```python
from build123d import *

# Parameters (mm, degrees)
F2_R     = 2
F3_DEPTH = 3
F4_R     = 1.5
F5_DEPTH = 8
F6_SIZE  = 0.2


with BuildPart() as f1:
    # F0 (on Right) → F1 (revolve)
    with BuildSketch(Plane.YZ):
        with BuildLine():
            Line((0, 3.25), (0, -3.25))
            ThreePointArc((0, -3.25), (3.25, 0), (0, 3.25))
        make_face()
    revolve(axis=Axis((0, 0, 0), (0, 0, -1)))

    # F2 (on Top) → F3 (join)
    with BuildSketch(Plane.XY):
        Circle(F2_R)
    extrude(amount=F3_DEPTH)

    # F4 (on face) → F5 (join)
    with BuildSketch(Plane.XY.offset(3)):
        Circle(F4_R)
    extrude(amount=F5_DEPTH)

    # F6
    f6_edges = [f1.edges().sort_by_distance(p)[0] for p in [
        (-1.5, 0, 11),
    ]]
    chamfer(f6_edges, length=F6_SIZE)


solid = f1.part
```
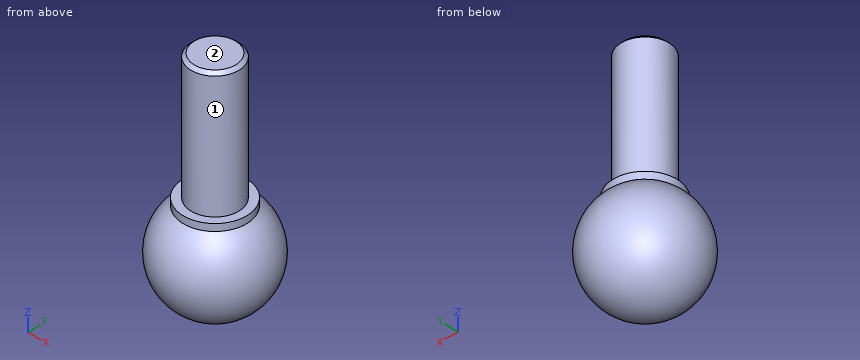
CAD build for the part. Positions are in the model's coordinates, mm. Face numbers are marked on the shaded views. A direction names the side the tool comes from. Give positions to 0.01 mm unless a question says otherwise; leave off trailing zeros. Write each loop counter-clockwise with the first axis right and the second up, starting at its lowest first coordinate (ties: lowest second). Pieces come first, ordered by that corner, then holes. Notation, with made-up numbers: M 69,21.5 L 113,21.5 A11 cw 113,29.5 Z; hole C 24,89 d7. An arc over 180 degrees is marked long. Return JSON: item names as keys, results as strings. Group by question number.
(1) 3-axis set-ups, long thin cutter, end or side, ignore diameter. For the marked faces 1 and 2: which of +Z, -Z, +X, -X, +Y, -Y reach the whole face in a straight line?
(2) Flat gauge pins, fed straight in: pin 1 Ø2 at (x, z) = (2, 9) entering from +Y; pin 2 Ø2 at (x, y) = (0, 1.5) entering from +Z. Where does each tip first touch, or does it go through?
(3) Band-saw the part on A-A (y = 0). Give the cut face in (x, z).
(4) Band-saw the part on D-D (z = 3.5). Give the cut face in (x, y).
(5) Band-saw the part on C-C (z = 1.25). Give the cut face in (x, y).
(6) Drill centre lines: L1, parallel to X at y = -0.25, z = 1.25; L2, parallel to X at y = 1, z = 2.75; L3, parallel to Y at x = 2, z = -2. Where is each one in solid material? Low to high. Write a range as [from, to].
Entries:
{
 "1": {"face 1": "+Z", "face 2": "+Z, +X, -X, +Y, -Y"},
 "2": {"pin 1": "stops at y = 1.12", "pin 2": "stops at z = 11"},
 "3": {"outline": "M -2,2.56 A3.25 ccw long 2,2.56 L 2,3 L 1.5,3 L 1.5,10.8 L 1.3,11 L -1.3,11 L -1.5,10.8 L -1.5,3 L -2,3 Z"},
 "4": {"outline": "C 0,0 d3"},
 "5": {"outline": "C 0,0 d6"},
 "6": {"L1": "x = [-2.99, 2.99]", "L2": "x = [-1.73, 1.73]", "L3": "y = [-1.6, 1.6]"}
}
